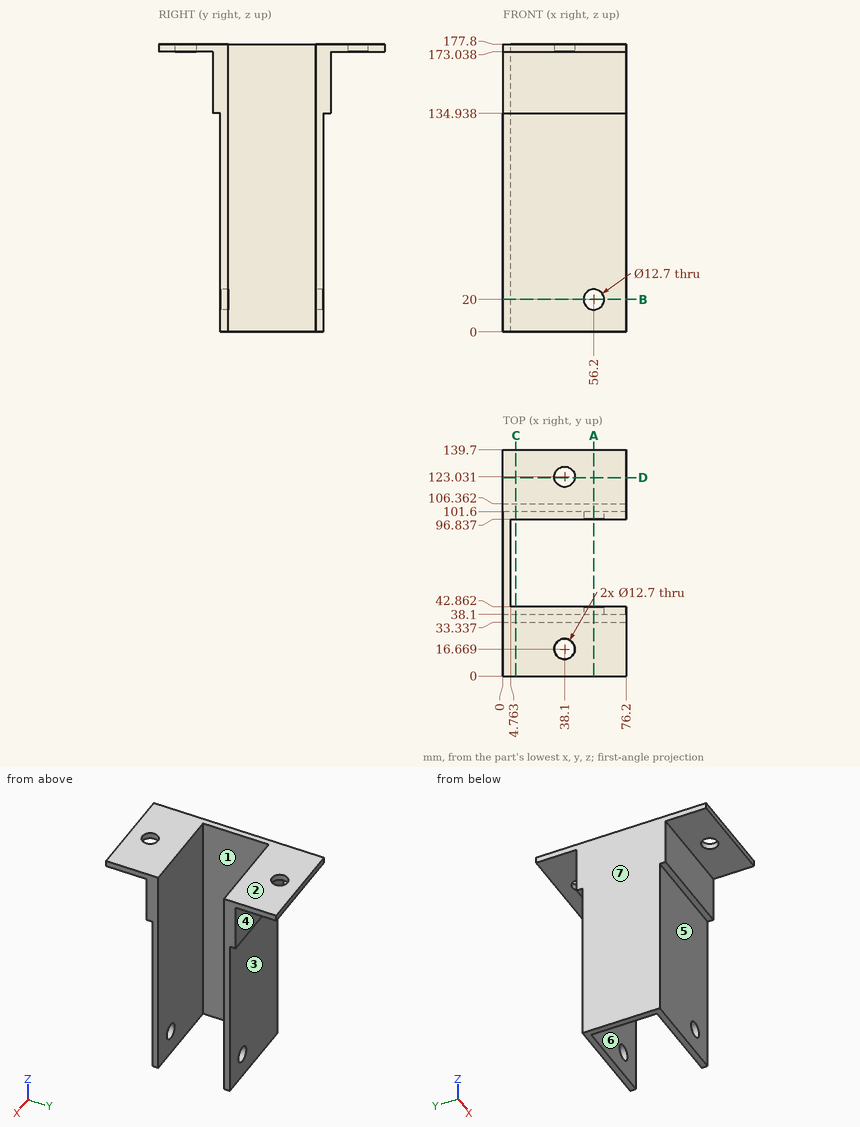
Design review of the part shown in the three views and the two pictorial views. Dimensions are in mm from the part's minimum x, y and z. A direction names the side the tool comes from. Give positions to 0.01 mm unless a question says otherwise; leave off trailing zeros. Write each loop counter-clockwise with the first axis right and the second up, starting at its lowest first coordinate (ties: lowest second). Pieces come first, ordered by that corner, then holes. Notation, with made-up numbers: (29.5, -18.75) -> (35.5, -18.75) arc R16 ccw to (35.5, -4.75) -> close; hole circle Ø5 at (31, 70.5). An arc over 180 degrees is marked (long way). Answer in a Markdown table with one row per item.
1) Clearance check with flat-ended pins moving along their axes: P1, Ø2.5, axis at x = 47.5, y = 36, coming from the -Z side; P2, Ø6, axis at x = 56, z = 72.5, coming from the -Y side; P3, Ø16.5, axis at x = 38.1, y = 123.03, coming from the -Z side; P4, Ø2, axis at y = 104.5, z = 28.5, coming from the -X side. State where each tip first meets the part, or that it passes through.
Worked answers:
| item | result |
|---|---|
| P1 | z = 134.94 |
| P2 | y = 38.1 |
| P3 | z = 173.04 |
| P4 | through |
2) Add section B-B on z = 20. State the section outline as (x, y) points.
Worked answers:
| item | result |
|---|---|
| outline | (0, 38.1) -> (49.85, 38.1) -> (49.85, 42.86) -> (4.76, 42.86) -> (4.76, 96.84) -> (49.85, 96.84) -> (49.85, 101.6) -> (0, 101.6) -> close; (62.55, 38.1) -> (76.2, 38.1) -> (76.2, 42.86) -> (62.55, 42.86) -> close; (62.55, 96.84) -> (76.2, 96.84) -> (76.2, 101.6) -> (62.55, 101.6) -> close |
3) Mouldability with a two-part tool opening along Y and no side actions: class the marked faces 1, 2 and 3 as +Y half, -Y half, draft (parallel to the pull), parting line (faces both ways), or undercut.
Worked answers:
| item | result |
|---|---|
| face 1 | undercut |
| face 2 | draft |
| face 3 | +Y half |
4) Tool access review of the marked faces 4, 5, 6 and 7: name each direction out of +Z, -Z, +X, -X, +Y, -Y from which nothing blocks a thin tool from reaching the whole face with its end or side.
Worked answers:
| item | result |
|---|---|
| face 4 | -Z, +X, -X, +Y |
| face 5 | -Z, +X, -X, -Y |
| face 6 | +Z, -Z, +X |
| face 7 | +Z, -Z, -X, +Y, -Y |
5) Add section A-A on x = 56.2. State the section outline as (y, z) points.
Worked answers:
| item | result |
|---|---|
| outline | (0, 173.04) -> (33.34, 173.04) -> (33.34, 134.94) -> (38.1, 134.94) -> (38.1, 26.35) -> (42.86, 26.35) -> (42.86, 177.8) -> (0, 177.8) -> close; (38.1, 0) -> (42.86, 0) -> (42.86, 13.65) -> (38.1, 13.65) -> close; (96.84, 0) -> (101.6, 0) -> (101.6, 13.65) -> (96.84, 13.65) -> close; (96.84, 26.35) -> (101.6, 26.35) -> (101.6, 134.94) -> (106.36, 134.94) -> (106.36, 173.04) -> (139.7, 173.04) -> (139.7, 177.8) -> (96.84, 177.8) -> close |
6) Add section D-D on y = 122.5. State the section outline as (x, z) points.
Worked answers:
| item | result |
|---|---|
| outline | (0, 173.04) -> (31.77, 173.04) -> (31.77, 177.8) -> (0, 177.8) -> close; (44.43, 173.04) -> (76.2, 173.04) -> (76.2, 177.8) -> (44.43, 177.8) -> close |
7) Add section C-C on x = 8. State the section outline as (y, z) points, plus the area to 3 significant figures.
Worked answers:
| item | result |
|---|---|
| outline | (0, 173.04) -> (33.34, 173.04) -> (33.34, 134.94) -> (38.1, 134.94) -> (38.1, 0) -> (42.86, 0) -> (42.86, 177.8) -> (0, 177.8) -> close; (96.84, 0) -> (101.6, 0) -> (101.6, 134.94) -> (106.36, 134.94) -> (106.36, 173.04) -> (139.7, 173.04) -> (139.7, 177.8) -> (96.84, 177.8) -> close |
| area | 2,420 mm² |
8) For L1, parallel to Y at x = 38, z = 174; L2, parallel to Y at x = 59.5, z = 34; L3, parallel to Y at x = 71.5, z = 148.5, list the stretches that pass through material, from the lowest coordinate up. Write a range as [from, to].
Worked answers:
| item | result |
|---|---|
| L1 | [0, 10.32], [23.02, 42.86], [96.84, 116.68], [129.38, 139.7] |
| L2 | [38.1, 42.86], [96.84, 101.6] |
| L3 | [33.34, 42.86], [96.84, 106.36] |
